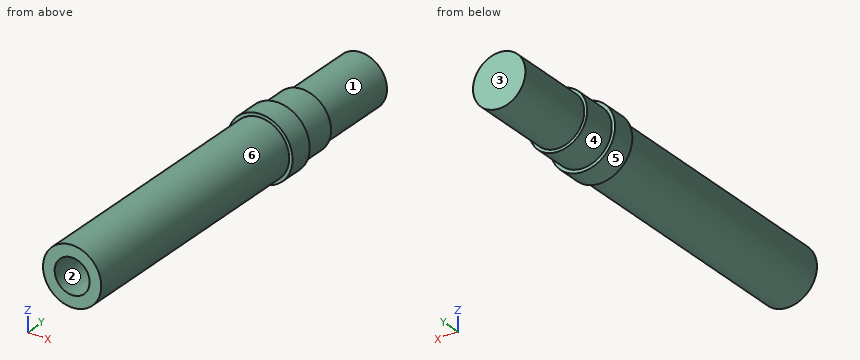
Autodesk Inventor part; units mm, degrees
ref_plane "YZ Plane" through (0, 0, 0) normal (1, 0, 0) x (0, 1, 0)
ref_plane "XZ Plane" through (0, 0, 0) normal (0, 1, 0) x (-1, 0, 0)
ref_plane "XY Plane" through (0, 0, 0) normal (0, 0, 1) x (1, 0, 0)
sketch "Sketch1" plane through (0, 0, 0) normal (0, 1, 0) x (-1, 0, 0)
  circle A0 centre (0, 0) radius 0.9525
  dimension "d0" = 1.905
extrude "Extrusion1" add sketch "Sketch1" along normal blind 8.7249
sketch "Sketch2" plane through (0, 8.7249, 0) normal (0, 1, 0) x (1, 0, 0)
  circle A0 centre (0, 0) radius 0.9525
  circle A1 centre (0, 0) radius 1.0605
  dimension "d3" = 2.1209
extrude "Extrusion2" add sketch "Sketch2" along normal blind 0.8001 contours A0 | A1
sketch "Sketch3" plane through (0, 9.525, 0) normal (0, 1, 0) x (1, 0, 0)
  circle A0 centre (0, 0) radius 1.0605
  circle A1 centre (0, 0) radius 0.9525
  circle A2 centre (0, 0) radius 0.8827
  dimension "d6" = 1.7653
extrude "Extrusion3" add sketch "Sketch3" along normal blind 1.143 contours A1 | A2
sketch "Sketch4" plane through (0, 10.668, 0) normal (0, 1, 0) x (1, 0, 0)
  circle A0 centre (0, 0) radius 0.9525
  circle A1 centre (0, 0) radius 0.8573
  dimension "d9" = 1.7145
extrude "Extrusion4" add sketch "Sketch4" along normal blind 2.7305 contours A1
sketch "Sketch5" plane through (0, 0, 0) normal (0, -1, 0) x (1, 0, 0)
  circle A0 centre (0, 0) radius 0.9525
  circle A1 centre (0, 0) radius 0.5715
  dimension "d12" = 1.143
extrude "Extrusion5" cut sketch "Sketch5" against normal blind 7.62 contours A1
properties part number "female_pin_component"
Design review of the part built by this model. Coordinates are the model's own, in mm. Face numbers are marked on the shaded views. A direction names the side the tool comes from. Round coordinates to 2 decimals unless told otherwise and drop trailing zeros. Loops run counter-clockwise (first coordinate to the right, second up) from the corner with the lowest first, then second, coordinate; pieces in that order, holes last. Notation, with made-up numbers: (50, 35.25) - (64, 35.25) arc R10 cw to (64, 53.25) - close; hole circle Ø6 at (-38, -6.5). An arc over 180 degrees is marked (long way). One line per item, written item: value. Start each with the question number.
1) Insertion check: pin 1 Ø0.7 at (x, z) = (0, 0) entering from -Y. The pin has a flat end and moves straight along its axis. Give the tip position at first contact, or say it passes through.
2) For the marked faces 4, 5 and 6, list the 3-axis set-ups (+Z, -Z, +X, -X, +Y, -Y) from which the entire face can be reached by the end or side of a thin tool; tool diameter is ignored.
3) Consider section D-D on y = 8.25. Give the boundary of the cut face in (x, z) (1 decimal).
4) To check wall thickness, follow L1, parallel to Z at x = 0, y = 5.25; L2, parallel to Y at x = 0.1, z = 0.45; L3, parallel to X at y = 1.25, z = 0.2. State the ranges of each line that lie inside material, in increasing order. Write a range as from..to.
5) Draft analysis for pull direction Z (two halves, no side actions). For the marked faces 1, 2 and 3, state which applies: +Z half, -Z half, draft (parallel to the pull), parting line (faces both ways), or undercut.
6) Consider section C-C on y = 4.5. Give the boundary of the cut face in (x, z) (1 decimal), then the cut area to 3 significant figures.
Reported:
1. pin 1: stops at y = 7.62
2. face 4: +Y
2. face 5: +Y, -Y
2. face 6: -Y
3. outline: circle Ø1.9 at (0, 0)
4. L1: z = -0.95..-0.57, 0.57..0.95
4. L2: y = 7.62..13.4
4. L3: x = -0.93..-0.54, 0.54..0.93
5. face 1: parting line
5. face 2: undercut
5. face 3: draft
6. outline: circle Ø1.9 at (0, 0); hole circle Ø1.1 at (0, 0)
6. area: 1.82 mm^2
